Drawing for the job (mm, zero at the part's lowest x, y, z). Coordinates: 2 decimals unless noted, no trailing zeros. Write each loop counter-clockwise with the first axis right and the second up, starting at its lowest first coordinate (ties: lowest second). Pieces come first, ordered by that corner, then holes.
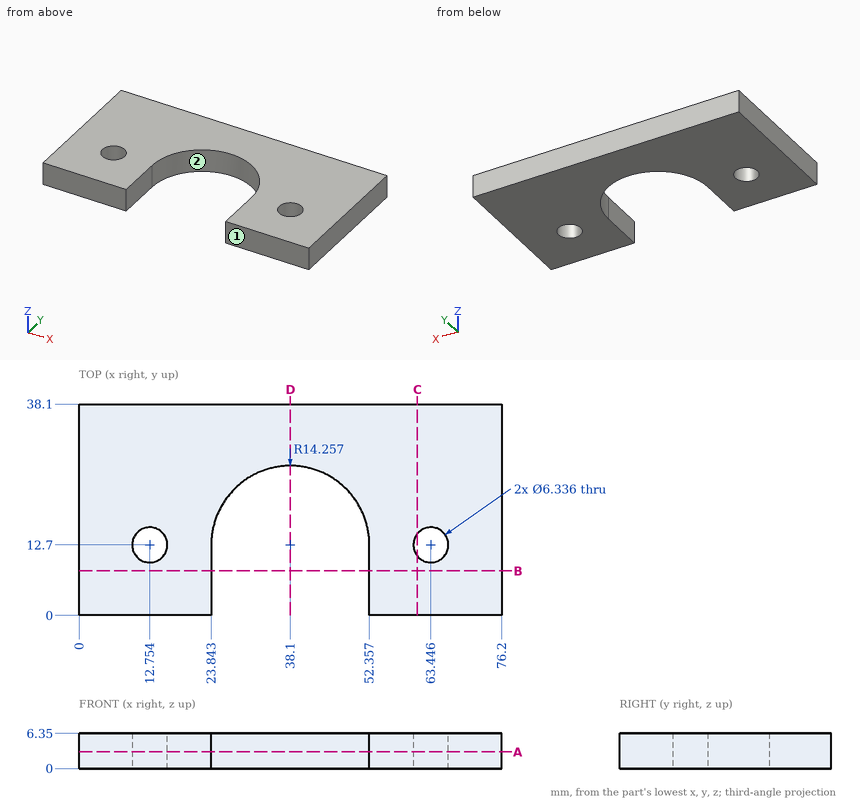
Item 1: Saw through at D-D, the plane x = 38.1. Write the cut outline in (y, z).
Item 2: Wall check: line 1 along X through (y, z) = (13, 4.75); line 2 along X through (y, z) = (11, 2); line 3 along Y through (x, z) = (66, 3.75) (1 decimal). Give the ranges that are in metal, low to high.
Item 3: Saw through at A-A, the plane z = 3. Write the cut outline in (x, y) (1 decimal).
Item 4: Saw through at C-C, the plane x = 61. Write the cut outline in (y, z), and give its area (3 significant figures).
Item 5: Saw through at B-B, the plane y = 8. Write the cut outline in (x, z), and give its area (3 significant figures).
Item 6: Two-plate mould, pull along X, no slides. Class the marked faces 1 and 2: +X half, -X half, draft (parallel to the pull), parting line (faces both ways), or undercut.
Working result:
1. outline: (26.96, 0) - (38.1, 0) - (38.1, 6.35) - (26.96, 6.35) - close
2. line 1: x = 0 to 9.6, 15.91 to 23.85, 52.35 to 60.29, 66.6 to 76.2
2. line 2: x = 0 to 10.08, 15.43 to 23.84, 52.36 to 60.77, 66.12 to 76.2
2. line 3: y = 0 to 10.8, 14.6 to 38.1
3. outline: (0, 0) - (23.8, 0) - (23.8, 12.7) arc R14.3 cw to (52.4, 12.7) - (52.4, 0) - (76.2, 0) - (76.2, 38.1) - (0, 38.1) - close; hole circle Ø6.3 at (12.8, 12.7); hole circle Ø6.3 at (63.4, 12.7)
4. outline: (0, 0) - (10.69, 0) - (10.69, 6.35) - (0, 6.35) - close; (14.71, 0) - (38.1, 0) - (38.1, 6.35) - (14.71, 6.35) - close
4. area: 216 mm2
5. outline: (0, 0) - (23.84, 0) - (23.84, 6.35) - (0, 6.35) - close; (52.36, 0) - (76.2, 0) - (76.2, 6.35) - (52.36, 6.35) - close
5. area: 303 mm2
6. face 1: draft
6. face 2: undercut
